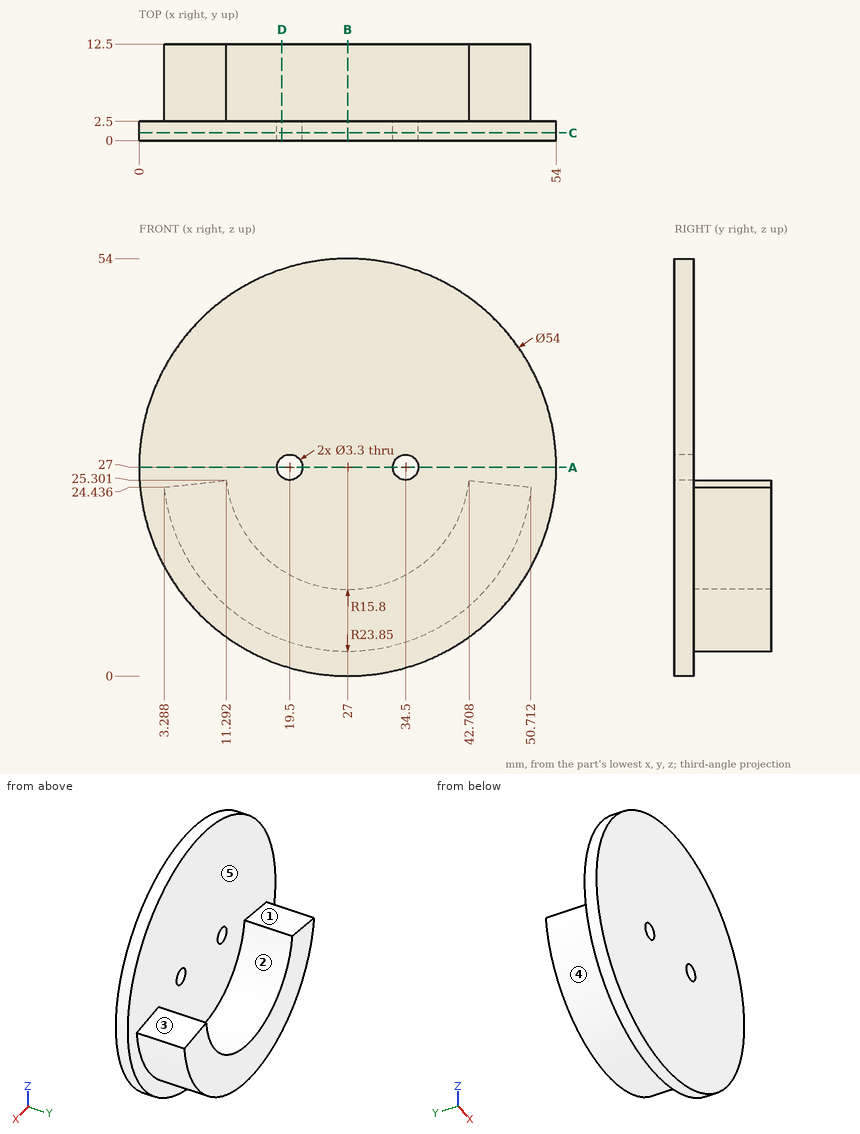
Check sheet for the drawn part. Datum: minimum x, y, z corner. Units: mm. A direction names the side the tool comes from. Round coordinates to 2 decimals unless told otherwise and drop trailing zeros. Order: outer loops, then holes, each group sorted by start corner. A loop starts at its lowest first (then second) coordinate and runs counter-clockwise, first axis right, second up. Notation, with made-up numbers: (-24, -37) -> (32, -37) arc R22 cw to (32, -19) -> close; hole circle Ø7 at (0, 55). An arc over 180 degrees is marked (long way). Return JSON: item names as keys, results as strings. Group by question number.
Q1. Tool access check on the marked faces 1, 2, 3, 4 and 5. Record the directions out of +Z, -Z, +X, -X, +Y, -Y that give a thin tool (end or side, any length) a straight path to the whole face; none if there is none.
Q2. Gauge pin test, flat ends, axial feed: pin 1 (6 mm diameter, centred on y = 7, z = 46, fed in from -X); pin 2 (6 mm diameter, centred on y = 3, z = 38.5, fed in from +X); pin 3 (16 mm diameter, centred on x = 39.5, z = 38.5, fed in from +Y); pin 4 (1.5 mm diameter, centred on x = 43.5, y = 2.5, fed in from +Z). Record the tip position at first contact, or that the pin passes through.
Q3. Section check B-B, the plane x = 27. Record the boundary of the cut face in (y, z).
Q4. Section check A-A, the plane z = 27. Record the boundary of the cut face in (x, y).
Q5. Material ranges on probe 1 along X at (y, z) = (1.6, 27); probe 2 along Y at (x, z) = (50, 41); probe 3 along X at (y, z) = (5.75, 17), recorded low to high. Write a range as from..to.
Q6. Section check C-C, the plane y = 1. Record the boundary of the cut face in (x, z).
Q7. Section check D-D, the plane x = 18.5. Record the boundary of the cut face in (y, z), plus the area to 3 significant figures.
Numbers:
{
 "1": {"face 1": "+Z, -X, +Y", "face 2": "+Z, +Y", "face 3": "+Z, +X, +Y", "face 4": "-Z, +Y", "face 5": "+Y"},
 "2": {"pin 1": "through", "pin 2": "x = 52.61", "pin 3": "y = 2.5", "pin 4": "z = 48.93"},
 "3": {"outline": "(0, 0) -> (2.5, 0) -> (2.5, 3.15) -> (12.5, 3.15) -> (12.5, 11.2) -> (2.5, 11.2) -> (2.5, 54) -> (0, 54) -> close"},
 "4": {"outline": "(0, 0) -> (17.85, 0) -> (17.85, 2.5) -> (0, 2.5) -> close; (21.15, 0) -> (32.85, 0) -> (32.85, 2.5) -> (21.15, 2.5) -> close; (36.15, 0) -> (54, 0) -> (54, 2.5) -> (36.15, 2.5) -> close"},
 "5": {"probe 1": "0..17.85, 21.15..32.85, 36.15..54", "probe 2": "0..2.5", "probe 3": "5.35..14.77, 39.23..48.65"},
 "6": {"outline": "circle Ø54 at (27, 27); hole circle Ø3.3 at (19.5, 27); hole circle Ø3.3 at (34.5, 27)"},
 "7": {"outline": "(0, 1.37) -> (2.5, 1.37) -> (2.5, 4.72) -> (12.5, 4.72) -> (12.5, 13.68) -> (2.5, 13.68) -> (2.5, 25.69) -> (0, 25.69) -> close; (0, 28.31) -> (2.5, 28.31) -> (2.5, 52.63) -> (0, 52.63) -> close", "area": "211 mm^2"}
}
